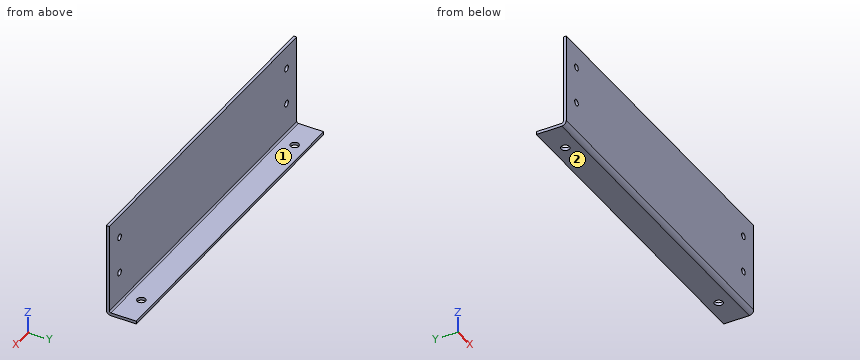
```python
from build123d import *

# Parameters (mm, degrees)
SKETCH_1_W             = 220
SKETCH_1_H             = 60
SM_BASE_FLANGE_1_DEPTH = 2
SM_EDGE_FLANGE_1_DEPTH = 220
MM_1_D                 = 5.5
MM_1_DEPTH             = 8
MM_1_TIP               = 1.652366702
HOLE_WIZARD_M5_1_D     = 4.2
HOLE_WIZARD_M5_1_DEPTH = 12.4
HOLE_WIZARD_M5_1_TIP   = 1.2618073


# Sheet-metal steps are written as plain solids
with BuildPart() as part:
    # Sketch 1 → 基体-法兰1 (new body)
    with BuildSketch(Plane(origin=(0, 0, 0), x_dir=(1, 0, 0), z_dir=(0, 1, 0))):
        with Locations((0, 30)):
            Rectangle(SKETCH_1_W, SKETCH_1_H)
    extrude(amount=-SM_BASE_FLANGE_1_DEPTH)

    # 边线-法兰1 section (across the edge) → 边线-法兰1 (add)
    with BuildSketch(Plane(origin=(110, 0, -61), x_dir=(0, 0, 1), z_dir=(-1, 0, 0))):
        with BuildLine():
            Line((-2, 1), (-2, 18))
            Line((-2, 18), (0, 18))
            Line((0, 18), (0, 1))
            ThreePointArc((0, 1), (0.292893219, 0.292893219), (1, 0))
            Line((1, 0), (1, -2))
            ThreePointArc((1, -2), (-1.121320344, -1.121320344), (-2, 1))
        make_face()
    extrude(amount=SM_EDGE_FLANGE_1_DEPTH)

    # 大小mm 暗销孔1
    with Locations(Plane(origin=(90, 10, -61), x_dir=(0, 1, 0), z_dir=(0, 0, 1))):
        with Locations((0, 0), (0, 180)):
            Hole(MM_1_D / 2, depth=MM_1_DEPTH)
            with Locations((0, 0, -(MM_1_DEPTH + MM_1_TIP / 2))):  # 118° drill point
                Cone(0, MM_1_D / 2, MM_1_TIP, mode=Mode.SUBTRACT)

    # M5 螺纹孔1
    with Locations(Plane(origin=(98, 0, -40), x_dir=(0, 0, 1), z_dir=(0, 1, 0))):
        with Locations((0, 0), (25, 0), (0, -196), (25, -196)):
            Hole(HOLE_WIZARD_M5_1_D / 2, depth=HOLE_WIZARD_M5_1_DEPTH)
            with Locations((0, 0, -(HOLE_WIZARD_M5_1_DEPTH + HOLE_WIZARD_M5_1_TIP / 2))):  # 118° drill point
                Cone(0, HOLE_WIZARD_M5_1_D / 2, HOLE_WIZARD_M5_1_TIP, mode=Mode.SUBTRACT)


solid = part.part
```
Verification items for the finished model (mm, model axes). Face numbers are marked on the shaded views. A direction names the side the tool comes from. Coordinates: 2 decimals unless noted, no trailing zeros. Order: outer loops, then holes, each group sorted by start corner. A loop starts at its lowest first (then second) coordinate and runs counter-clockwise, first axis right, second up. Notation, with made-up numbers: (65, 59.25) -> (72, 59.25) arc R21 ccw to (72, 86.25) -> close; hole circle Ø2 at (-6, -24). An arc over 180 degrees is marked (long way). Answer as CSV lines item,"result". Start each with the question number.
1) Cross-section at D-D, the plane x = -98. Record the boundary of the cut face in (y, z), then the cut area to 3 significant figures.
2) Cross-section at C-C, the plane y = 10. Record the boundary of the cut face in (x, z).
3) Material ranges on L1, parallel to X at y = -1.1, z = -15; L2, parallel to X at y = 10, z = -61.7; L3, parallel to Y at x = 13, z = -40, recorded low to high. Write a range as [from, to].
4) Gauge pin test, flat ends, axial feed: pin 1 Ø12 at (x, y) = (-3, 12) entering from +Z; pin 2 Ø12 at (x, z) = (48, -23) entering from +Y. Record the tip position at first contact, or that the pin passes through.
5) Cross-section at B-B, the plane z = -15. Record the boundary of the cut face in (x, y), then the cut area to 3 significant figures.
6) Cross-section at A-A, the plane x = 90. Record the boundary of the cut face in (y, z).
7) Set-up check for the marked faces 1 and 2: record each of +Z, -Z, +X, -X, +Y, -Y from which the full face is reachable in a straight line by a thin tool's end or side.
Conclusion:
1,outline,"(-2, -60) arc R3 ccw to (1, -63) -> (18, -63) -> (18, -61) -> (1, -61) arc R1 cw to (0, -60) -> (0, -42.1) -> (-2, -42.1) -> close; (-2, -37.9) -> (0, -37.9) -> (0, -17.1) -> (-2, -17.1) -> close; (-2, -12.9) -> (0, -12.9) -> (0, 0) -> (-2, 0) -> close"
1,area,"143 mm²"
2,outline,"(-110, -63) -> (-92.75, -63) -> (-92.75, -61) -> (-110, -61) -> close; (-87.25, -63) -> (87.25, -63) -> (87.25, -61) -> (-87.25, -61) -> close; (92.75, -63) -> (110, -63) -> (110, -61) -> (92.75, -61) -> close"
3,L1,"x = [-110, -100.1], [-95.9, 95.9], [100.1, 110]"
3,L2,"x = [-110, -92.75], [-87.25, 87.25], [92.75, 110]"
3,L3,"y = [-2, 0]"
4,pin 1,"stops at z = -61"
4,pin 2,"stops at y = 0"
5,outline,"(-110, -2) -> (-100.1, -2) -> (-100.1, 0) -> (-110, 0) -> close; (-95.9, -2) -> (95.9, -2) -> (95.9, 0) -> (-95.9, 0) -> close; (100.1, -2) -> (110, -2) -> (110, 0) -> (100.1, 0) -> close"
5,area,"423 mm²"
6,outline,"(-2, -60) arc R3 ccw to (1, -63) -> (7.25, -63) -> (7.25, -61) -> (1, -61) arc R1 cw to (0, -60) -> (0, 0) -> (-2, 0) -> close; (12.75, -63) -> (18, -63) -> (18, -61) -> (12.75, -61) -> close"
7,face 1,"+Z, +X, -X, +Y"
7,face 2,"-Z, +X, -X, +Y, -Y"
